Model file for the job. Use its own axes, mm. A direction names the side the tool comes from. Round coordinates to 2 decimals unless told otherwise and drop trailing zeros. Order: outer loops, then holes, each group sorted by start corner. A loop starts at its lowest first (then second) coordinate and runs counter-clockwise, first axis right, second up. Notation, with made-up numbers: (45.5, 51) - (87.5, 51) arc R24 cw to (87.5, 82) - close; hole circle Ø4 at (58.25, 23.5). An arc over 180 degrees is marked (long way). Put each result on its own line as item: value. Start each with the question number.
Item 1: Saw through at B-B on z = 25. List the corners of the cut face in (x, y), plus the area to 3 significant figures.
Item 2: Probe probe 1 along Z at (x, y) = (24.5, 11); probe 2 along X at (y, z) = (0.9, 25). List the from-to ranges inside material, lowest first.
Item 3: Saw through at A-A on x = 25. List the corners of the cut face in (y, z), plus the area to 3 significant figures.
Item 4: Pin check, flat tip, straight feed: pin 1 Ø6 at (x, z) = (43, 42) entering from +Y. Stop position of the tip, or through.
Item 5: Saw through at C-C on y = 49. List the corners of the cut face in (x, z), plus the area to 3 significant figures.
Item 6: Which spindle directions (+Z, -Z, +X, -X, +Y, -Y) get a long thin tool onto all of the face, cutting with end or side? Do faces 1 (the face through (3, 37, 25)), 2 (the face through (0.86, 36.5, 49.1)). Say none if no direction does.
Item 7: Saw through at D-D on z = 39. List the corners of the cut face in (x, y).
Item 8: Mould opens along Z. For faces 3 (the face through (47, 37, 25)), 4 (the face through (49.14, 36.5, 0.9)), 5 (the face through (0, 35, 25)) say: pulls with the +Z half, pulls with the -Z half, needs draft (parallel to the pull), parting line crosses it, or undercut.
```python
from build123d import *

# Parameters (mm, degrees)
SKETCH_1_W              = 50
SKETCH_1_H              = 72
STEPPER_COVER_DEPTH     = 50
FILLET_2_R              = 3
SHELL_START             = 3
SHELL_1_OUTLINE_W       = 69
SHELL_1_OUTLINE_H       = 44
SHELL_1_DEPTH           = 44
SKETCH_2_R              = 12
COUPLER_CLEARANCE_DEPTH = 3.1


# Read off the part's stored shape, not the designer's step: 抽壳1
with BuildPart() as part:
    # 草图1 → Stepper_cover (new body)
    with BuildSketch(Plane.XY):
        with Locations((25, 36)):
            Rectangle(SKETCH_1_W, SKETCH_1_H)
    extrude(amount=STEPPER_COVER_DEPTH)

    # Fillet 2
    fillet_2_edges = [part.edges().sort_by_distance(p)[0] for p in [
        (50, 36, 50),
        (0, 36, 50),
        (50, 36, 0),
        (0, 36, 0),
    ]]
    fillet(fillet_2_edges, radius=FILLET_2_R)

    # 抽壳1 outline → 抽壳1 (cut)
    with BuildSketch(Plane.YZ.offset(SHELL_START)):
        with Locations((37.5, 25)):
            Rectangle(SHELL_1_OUTLINE_W, SHELL_1_OUTLINE_H)
    extrude(amount=SHELL_1_DEPTH, mode=Mode.SUBTRACT)

    # 草图2 → Coupler_clearance (cut)
    with BuildSketch(Plane.XZ):
        with Locations(Location((25, 25, 0), (0, 0, 270))):
            Circle(SKETCH_2_R)
    extrude(amount=-COUPLER_CLEARANCE_DEPTH, mode=Mode.SUBTRACT)


solid = part.part
```
Results found:
1. outline: (0, 0) - (13, 0) - (13, 3) - (3, 3) - (3, 72) - (0, 72) - close; (37, 0) - (50, 0) - (50, 72) - (47, 72) - (47, 3) - (37, 3) - close
1. area: 492 mm²
2. probe 1: z = 0 to 3, 47 to 50
2. probe 2: x = 0 to 13, 37 to 50
3. outline: (0, 0) - (72, 0) - (72, 3) - (3, 3) - (3, 13) - (0, 13) - close; (0, 37) - (3, 37) - (3, 47) - (72, 47) - (72, 50) - (0, 50) - close
3. area: 492 mm²
4. pin 1: stops at y = 3
5. outline: (0, 3) arc R3 ccw to (3, 0) - (47, 0) arc R3 ccw to (50, 3) - (50, 47) arc R3 ccw to (47, 50) - (3, 50) arc R3 ccw to (0, 47) - close; hole (3, 3) - (47, 3) - (47, 47) - (3, 47) - close
5. area: 556 mm²
6. face 1: +Y
6. face 2: +Z, -X, +Y, -Y
7. outline: (0, 0) - (50, 0) - (50, 72) - (47, 72) - (47, 3) - (3, 3) - (3, 72) - (0, 72) - close
8. face 3: undercut
8. face 4: pulls with the -Z half
8. face 5: needs draft
